Here's how the part is built. I have some questions about the finished solid (model axes, mm). Face numbers are marked on the shaded views. A direction names the side the tool comes from. Round coordinates to 2 decimals unless told otherwise and drop trailing zeros. Order: outer loops, then holes, each group sorted by start corner. A loop starts at its lowest first (then second) coordinate and runs counter-clockwise, first axis right, second up. Notation, with made-up numbers: (15.5, 44) -> (59.5, 44) arc R30 cw to (59.5, 66) -> close; hole circle Ø4 at (88, 37.25). An arc over 180 degrees is marked (long way). Use a Markdown table: item, result. Add a question column.
(1) I want a section at A-A, the plane x = 44. Please give me the cut outline in (y, z), then the cut area to 3 significant figures.
(2) If I drill on probe 1 along Y at (x, z) = (0.5, 1.2); probe 2 along Y at (x, z) = (55, 0.4); probe 3 along X at (y, z) = (6.5, 1.5), over which ranges is the centre line in solid material (lowest first)?
(3) I want a section at D-D, the plane x = 52. Please give me the cut outline in (y, z).
(4) I'm going to push flat-ended pins straight in: P1, Ø2, axis at y = 23, z = 2, coming from the +X side; P2, Ø2, axis at y = 18.5, z = 3, coming from the -X side. Where does each tip first touch, or does it pass through?
(5) On a 3-axis mill with a long thin cutter (end or side, diameter ignored), from which of +Z, -Z, +X, -X, +Y, -Y can I reach the whole of each face in a straight line? I mean the marked faces 5, 6 and 7. Say none if no direction works.
(6) I want a section at C-C, the plane z = 1.35. Please give me the cut outline in (x, y), then the cut area to 3 significant figures.
(7) Thinking about a two-plate mould opening in Y: for the marked faces 1, 2, 3 and 4, which applies, pulls with the +Y half, pulls with the -Y half, needs draft (parallel to the pull), parting line crosses it, or undercut?
(8) I want a section at B-B, the plane y = 11.5. Please give me the cut outline in (x, z), then the cut area to 3 significant figures.
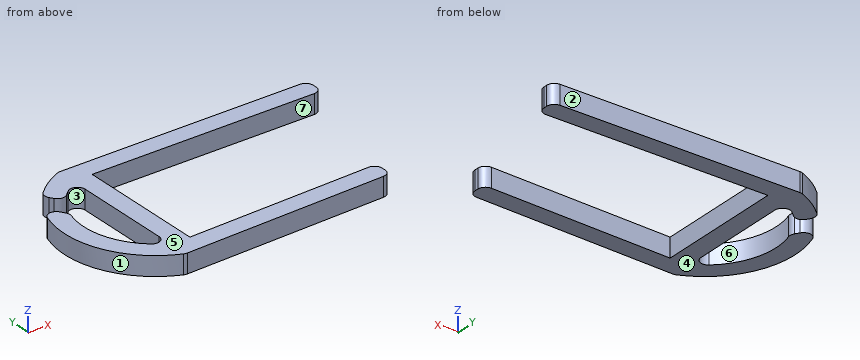
from build123d import *

# Parameters (mm, degrees)
F1_DEPTH = 5
F2_R     = 2


with BuildPart() as f1:
    # F0 (on Top) → F1 (new body)
    with BuildSketch(Plane.XY):
        Polygon((49.969541351, 1.7449748351), (0, 0), (0, 33.9), (60, 33.9), (60, 38.9), (-5, 38.9), (-5, 33.4082755117), (-5, 0.3140729194), (-5, -5.177651569), (49.969541351, -3.2580728864), align=None)
        with BuildLine():
            Line((-5, 33.4082755117), (-5, 38.9))
            ThreePointArc((-5, 38.9), (-9.8858414628, 36.2755829056), (-14.0276237399, 32.5871345254))
            Line((-14.0276237399, 32.5871345254), (-11.1949861447, 28.1640846398))
            ThreePointArc((-11.1949861447, 28.1640846398), (-8.385603023, 31.1265256497), (-5, 33.4082755117))
        make_face()
        with BuildLine():
            ThreePointArc((-17.1309979161, 28.161794916), (-18.5720640821, 8.7607088143), (-5, -5.177651569))
            Line((-5, -5.177651569), (-5, 0.3140729194))
            ThreePointArc((-5, 0.3140729194), (-13.7193681247, 10.061847649), (-13.9141851806, 23.1388709719))
            Line((-13.9141851806, 23.1388709719), (-17.1309979161, 28.161794916))
        make_face()
    extrude(amount=F1_DEPTH)

    # F2
    f2_edges = [f1.edges().sort_by_distance(p)[0] for p in [
        (49.969541, 1.744975, 2.5),
        (49.969541, -3.258073, 2.5),
        (-5, -5.177652, 2.5),
        (-5, 0.314073, 2.5),
        (-5, 33.408276, 2.5),
        (60, 33.9, 2.5),
        (-17.130998, 28.161795, 2.5),
        (-14.027624, 32.587135, 2.5),
        (-13.914185, 23.138871, 2.5),
        (-11.194986, 28.164085, 2.5),
        (-5, 38.9, 2.5),
        (60, 38.9, 2.5),
    ]]
    fillet(f2_edges, radius=F2_R)


solid = f1.part
Taken from the geometry:
| question | item | result |
|---|---|---|
| 1 | outline | (-3.47, 0) -> (1.54, 0) -> (1.54, 5) -> (-3.47, 5) -> close; (33.9, 0) -> (38.9, 0) -> (38.9, 5) -> (33.9, 5) -> close |
| 1 | area | 50.0 mm2 |
| 2 | probe 1 | y = -4.99 to 0.02, 33.9 to 38.9 |
| 2 | probe 2 | y = 33.9 to 38.9 |
| 2 | probe 3 | x = -17.61 to -11.87, -5 to 0 |
| 3 | outline | (33.9, 0) -> (38.9, 0) -> (38.9, 5) -> (33.9, 5) -> close |
| 4 | P1 | stops at x = 0 |
| 4 | P2 | stops at x = -19.99 |
| 5 | face 5 | +Z, +X, -X, +Y, -Y |
| 5 | face 6 | +Z, -Z |
| 5 | face 7 | +Z, -Z, +X |
| 6 | outline | (-18.7, 24.6) arc R23.69 ccw to (-5.41, -5.01) arc R2 ccw to (-4.57, -5.16) -> (48.04, -3.33) arc R2 ccw to (49.97, -1.33) -> (49.97, -0.33) arc R2 ccw to (47.9, 1.67) -> (0, 0) -> (0, 33.9) -> (58, 33.9) arc R2 ccw to (60, 35.9) -> (60, 36.9) arc R2 ccw to (58, 38.9) -> (-4.61, 38.9) arc R2 ccw to (-5.38, 38.75) arc R23.69 ccw to (-12.9, 33.77) arc R2 ccw to (-13.18, 31.27) -> (-12.63, 30.41) arc R2 ccw to (-9.53, 30.07) arc R18.69 cw to (-8.28, 31.21) arc R2 cw to (-5, 29.68) -> (-5, 4.04) arc R2 cw to (-8.28, 2.51) arc R18.69 cw to (-14.2, 22.28) arc R2 ccw to (-14.43, 23.94) -> (-15.12, 25.03) arc R2 ccw to start |
| 6 | area | 983 mm2 |
| 7 | face 1 | parting line crosses it |
| 7 | face 2 | pulls with the +Y half |
| 7 | face 3 | undercut |
| 7 | face 4 | needs draft |
| 8 | outline | (-19.39, 0) -> (-14.21, 0) -> (-14.21, 5) -> (-19.39, 5) -> close; (-5, 0) -> (0, 0) -> (0, 5) -> (-5, 5) -> close |
| 8 | area | 50.9 mm2 |
